from build123d import *

# Parameters (mm, degrees)
F0_R     = 21.59
F0_R_2   = 17.526
F1_DEPTH = 18.796
F2_R     = 1.397
F3_DEPTH = 5.334
F5_DEPTH = 5.32335


# Not quite as in the source:
# - a fillet or chamfer that OpenCascade refuses, or shapes differently, is made with other operations: its cross-section is extruded or revolved along the edge and cut away or added


with BuildPart() as f1:
    # F0 (on Top) → F1 (new body)
    with BuildSketch(Plane.XY):
        Circle(F0_R)
        Circle(F0_R_2, mode=Mode.SUBTRACT)
    extrude(amount=F1_DEPTH)

    # F2 (on face) → F3 (join)
    with BuildSketch(Plane(origin=(0, 0, 0), x_dir=(1, 0, 0), z_dir=(0, 0, -1))):
        with BuildLine():
            ThreePointArc((-21.2075058824, -4.0459602383), (-21.5081828799, 0), (-21.2075058824, 4.0459602383))
            ThreePointArc((-21.2075058824, 4.0459602383), (-25.5653001948, 0), (-21.2075058824, -4.0459602383))
        make_face()
        with Locations((-23.622, 0)):
            Circle(F2_R, mode=Mode.SUBTRACT)
        with BuildLine():
            ThreePointArc((-4.0459602383, 21.2075058824), (0, 21.59), (4.0459602383, 21.2075058824))
            ThreePointArc((4.0459602383, 21.2075058824), (0, 25.6437689885), (-4.0459602383, 21.2075058824))
        make_face()
        with Locations((0, 23.622)):
            Circle(F2_R, mode=Mode.SUBTRACT)
    extrude(amount=-F3_DEPTH)

    # F4 (on face) → F5 (join)
    with BuildSketch(Plane.XY.offset(5.334)):
        with BuildLine():
            ThreePointArc((15.2619734187, 15.2619734187), (16.6668392005, 13.6913700024), (17.9108306766, 11.990508996))
            ThreePointArc((17.9108306766, 11.990508996), (19.4564957211, 15.0391701429), (18.2294215901, 18.2294215901))
            Line((18.2294215901, 18.2294215901), (17.6633479303, 17.6633479303))
            ThreePointArc((17.6633479303, 17.6633479303), (17.9661794639, 17.210128512), (18.072519757, 16.675519757))
            ThreePointArc((18.072519757, 16.675519757), (17.210128512, 15.3848600501), (15.6876915837, 15.6876915837))
            Line((15.6876915837, 15.6876915837), (15.2619734187, 15.2619734187))
        make_face()
        with BuildLine():
            Line((17.6633479303, 17.6633479303), (18.2294215901, 18.2294215901))
            ThreePointArc((18.2294215901, 18.2294215901), (15.0665422687, 19.4578041419), (12.025389791, 17.9531045364))
            ThreePointArc((12.025389791, 17.9531045364), (13.7098474372, 16.6871156464), (15.2619734187, 15.2619734187))
            Line((15.2619734187, 15.2619734187), (15.6876915837, 15.6876915837))
            ThreePointArc((15.6876915837, 15.6876915837), (15.6876915837, 17.6633479303), (17.6633479303, 17.6633479303))
        make_face()
    extrude(amount=-F5_DEPTH)

    # F6: fillet of radius 5.08 on 1 edges, made by hand

    # F6_s1 → F6_t2 (revolve, cut)
    with BuildSketch(Plane.XZ):
        with BuildLine():
            ThreePointArc((21.59, 13.8186368427), (20.4449510797, 17.0315109454), (17.526, 18.796))
            Line((17.526, 18.796), (21.59, 18.796))
            Line((21.59, 18.796), (21.59, 13.8186368427))
        make_face()
    revolve(axis=Axis((0, 0, 18.796), (0, 0, 1)), mode=Mode.SUBTRACT)


solid = f1.part
Design review of the part built by this model. Coordinates are the model's own, in mm. A direction names the side the tool comes from. Coordinates: 2 decimals unless noted, no trailing zeros. Order: outer loops, then holes, each group sorted by start corner. A loop starts at its lowest first (then second) coordinate and runs counter-clockwise, first axis right, second up. Notation, with made-up numbers: M 67.25,55 L 126.25,55 A17 cw 126.25,60 Z; hole C 55,-7.5 d1. An arc over 180 degrees is marked long. Use a Markdown table: item, result.
(1) Add section D-D (x = 16.5). Count the separate pieces of the cut face and the enclosed holes in it, then the cut area to 3 significant figures.
Worked answers:
| item | result |
|---|---|
| separate pieces | 3 |
| enclosed holes | 0 |
| area | 298 mm2 |
(2) Draft analysis for pull direction X (two halves, no side actions). For faces 1 (the cylindrical face through (0.095, -25.643, 2.63)), 2 (the flat face through (-22, 1, 5.334)), 3 (the cylindrical face through (-0.303, -22.258, 2.63)), state which applies: released by +X, released by -X, zero draft, split by the parting line, or undercut.
Worked answers:
| item | result |
|---|---|
| face 1 | split by the parting line |
| face 2 | zero draft |
| face 3 | undercut |
(3) For P1, Ø3, axis at x = -7.5, z = 10, coming from the -Y side; P2, Ø5, axis at x = -22.5, y = -1, coming from the +Z side; P3, Ø10, axis at x = -10.5, y = -15.5, coming from the -Z side; P4, Ø5, axis at x = 12.5, z = 8.5, coming from the -Y side, all flat-tipped, find the tip position at first contact; note any pin that passes through.
Worked answers:
| item | result |
|---|---|
| P1 | stops at y = -20.74 |
| P2 | stops at z = 17.49 |
| P3 | stops at z = 0 |
| P4 | stops at y = -19.13 |
(4) Add section B-B (y = 0). Give the boundary of the cut face in (x, z) (3 decimals), then the cut area to 3 significant figures.
Worked answers:
| item | result |
|---|---|
| outline | M -25.565,0 L -25.019,0 L -25.019,5.334 L -25.565,5.334 Z; M -22.225,0 L -17.526,0 L -17.526,18.796 A5.08 ccw -21.59,13.819 L -21.59,5.334 L -22.225,5.334 Z; M 17.526,0 L 21.59,0 L 21.59,13.819 A5.08 ccw 17.526,18.796 Z |
| area | 149 mm2 |
(5) Wall thickness on probe 1 along Y at (x, z) = (0, 3.25) (3 decimals); probe 2 along Y at (x, z) = (0, 9); probe 3 along Z at (x, y) = (-3, -20.5): over which ranges is each line inside the solid? List them lowest first.
Worked answers:
| item | result |
|---|---|
| probe 1 | y = -25.644 to -25.019, -22.225 to -17.526, 17.526 to 21.59 |
| probe 2 | y = -21.59 to -17.53, 17.53 to 21.59 |
| probe 3 | z = 0 to 16.66 |
(6) Add section C-C (z = 17.5). Give the boundary of the cut face in (x, y).
Worked answers:
| item | result |
|---|---|
| outline | C 0,0 d40.02; hole C 0,0 d35.05 |
(7) For faces 4 (the flat face through (15, 17, 5.334)), 5 (the flat face through (-18, 0, 0)), list the 3-axis set-ups (+Z, -Z, +X, -X, +Y, -Y) from which the entire face can be reached by the end or side of a thin tool; tool diameter is ignored.
Worked answers:
| item | result |
|---|---|
| face 4 | +Z, +X, +Y |
| face 5 | -Z, +X, -X, +Y, -Y |
(8) Add section A-A (x = 0). Give the boundary of the cut face in (y, z) (3 decimals).
Worked answers:
| item | result |
|---|---|
| outline | M -25.644,0 L -25.019,0 L -25.019,5.334 L -25.644,5.334 Z; M -22.225,0 L -17.526,0 L -17.526,18.796 A5.08 ccw -21.59,13.819 L -21.59,5.334 L -22.225,5.334 Z; M 17.526,0 L 21.59,0 L 21.59,13.819 A5.08 ccw 17.526,18.796 Z |
